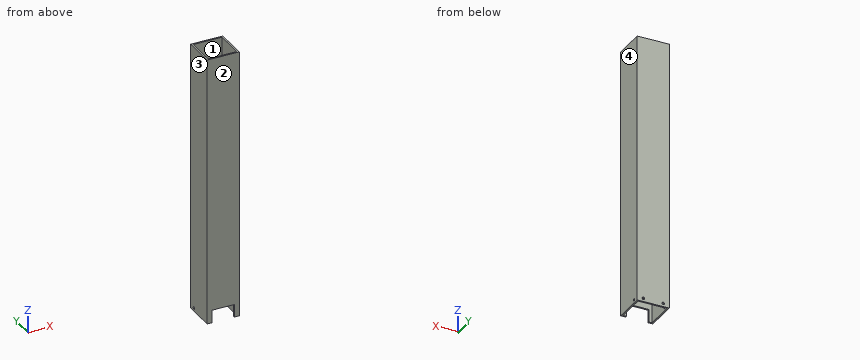
Autodesk Inventor part; units mm, degrees
ref_plane "YZ Plane" through (0, 0, 0) normal (1, 0, 0) x (0, 1, 0)
ref_plane "XZ Plane" through (0, 0, 0) normal (0, 1, 0) x (-1, 0, 0)
ref_plane "XY Plane" through (0, 0, 0) normal (0, 0, 1) x (1, 0, 0)
sketch "Sketch1" plane through (0, 0, 0) normal (0, 0, 1) x (1, 0, 0)
  line L0 (0, 0) -> (63.5, 0)
  line L1 (63.5, 0) -> (63.5, 63.5)
  line L2 (63.5, 63.5) -> (0, 63.5)
  line L3 (0, 63.5) -> (0, 0)
  line L4 (3.175, 60.325) -> (60.325, 60.325)
  line L5 (60.325, 60.325) -> (60.325, 3.175)
  line L6 (60.325, 3.175) -> (3.175, 3.175)
  line L7 (3.175, 3.175) -> (3.175, 60.325)
  dimension "d0" = 63.5
  dimension "d1" = 63.5
  dimension "d2" = 3.175
extrude "Extrusion1" add sketch "Sketch1" along normal blind 533.4
sketch "Sketch3" plane through (0, 63.5, 0) normal (0, 1, 0) x (1, 0, 0)
  line L0 (9.525, 0) -> (9.525, -25.4)
  line L1 (9.525, -25.4) -> (53.975, -25.4)
  line L2 (53.975, -25.4) -> (53.975, 0)
  line L3 (63.5, 0) -> (63.5, -533.4)
  line L4 (63.5, 0) -> (0, 0)
  line L5 (9.525, 0) -> (53.975, 0)
  line L6 (0, 0) -> (63.5, 0)
  line L7 (63.5, 0) -> (0, 0)
  line L8 (0, 0) -> (0, -533.4)
  line L9 (63.5, -533.4) -> (0, -533.4)
  line L10 (63.5, 0) -> (63.5, -533.4)
  dimension "d14" = 44.45
  dimension "d16" = 25.4
  dimension "d19" = 9.525
  dimension "d20" = 9.525
extrude "Extrusion2" cut sketch "Sketch3" against normal blind 63.5 contours L4 L2 L1 L0
sketch "Sketch5" plane through (0, 63.5, 533.4) normal (0, 1, 0) x (1, 0, 0)
  line L0 (53.975, 508) -> (9.525, 508)
  line L1 (53.975, 533.4) -> (53.975, 508)
  line L2 (9.525, 508) -> (9.525, 533.4)
  line L3 (53.975, 533.4) -> (9.525, 533.4)
  point P0 (0, 533.4)
extrude "Extrusion3" add sketch "Sketch5" against normal blind 3.175
sketch "Sketch6" plane through (0, 63.5, 0) normal (0, 1, 0) x (1, 0, 0)
  line L0 (0, 0) -> (0, -533.4)
  line L1 (63.5, 0) -> (63.5, -533.4)
  line L2 (63.5, 0) -> (0, 0)
  point P0 (12.192, -6.35)
  point P1 (51.308, -6.35)
  dimension "d23" = 12.192
  dimension "d24" = 12.192
  dimension "d25" = 6.35
hole "Hole2" at (12.192, 63.5, 6.35) at (51.308, 63.5, 6.35) direction (0, -1, 0) diameter 5.1562 depth 25.4 tip angle 118
sketch "Sketch7" plane through (63.5, 0, 0) normal (1, 0, 0) x (0, 0, -1)
  line L0 (0, 63.5) -> (-533.4, 63.5)
  line L1 (0, 0) -> (0, 63.5)
  point P0 (-6.35, 51.308)
  dimension "d33" = 12.192
  dimension "d34" = 6.35
hole "Hole3" at (63.5, 51.308, 6.35) direction (-1, 0, 0) diameter 5.1562 depth 76.2 tip angle 118
equation "\"d19\" = d20"
properties part number "TelescopeNewOuter" material "Aluminum 6061"
The listing builds one solid part. Answer for the finished solid, in the listing's coordinates (mm). Face numbers are marked on the shaded views. Round coordinates to 2 decimals unless told otherwise and drop trailing zeros. Write each loop counter-clockwise with the first axis right and the second up, starting at its lowest first coordinate (ties: lowest second). Pieces come first, ordered by that corner, then holes. Notation, with made-up numbers: (60.5, 15.5) -> (87.5, 15.5) arc R27 cw to (87.5, 43.5) -> close; hole circle Ø8 at (-11.75, 38.25). An arc over 180 degrees is marked (long way). Use CSV: the item, a comma, the result in double quotes. Start each with the question number.
(1) The mould has two halves that part along X. Classify the marked faces 1, 2, 3 and 4: released by +X, released by -X, zero draft, split by the parting line, or undercut.
(2) Consider L1, parallel to X at y = 61.65, z = 6.35; L2, parallel to Y at x = 60, z = 314 (3 decimals). Determine where each line is inside the solid, lowest interval first. Write a range as from..to.
(3) This flat-tipped pin is pushed along its axis until it touches: pin 1 (2.5 mm diameter, centred on x = 28.5, y = 1, fed in from -Z). Where does it stop, or does it pass through?
(4) Section B-B on z = 465 is taken. Give the vertices of the cut face in (x, y) (3 decimals), then the cut area to 3 significant figures.
(5) Section A-A on y = 31 is taken. Give the vertices of the cut face in (x, z) (3 decimals), then the cut area to 3 significant figures.
(6) Section C-C on x = 30 is taken. Give the vertices of the cut face in (y, z) (3 decimals), then the cut area to 3 significant figures.
A:
1,face 1,"undercut"
1,face 2,"zero draft"
1,face 3,"released by -X"
1,face 4,"released by +X"
2,L1,"x = 0..9.61, 14.77..48.73, 53.89..63.5"
2,L2,"y = 0..3.175, 60.325..63.5"
3,pin 1,"stops at z = 25.4"
4,outline,"(0, 0) -> (63.5, 0) -> (63.5, 63.5) -> (0, 63.5) -> close; hole (3.175, 3.175) -> (60.325, 3.175) -> (60.325, 60.325) -> (3.175, 60.325) -> close"
4,area,"766 mm²"
5,outline,"(0, 0) -> (3.175, 0) -> (3.175, 533.4) -> (0, 533.4) -> close; (60.325, 0) -> (63.5, 0) -> (63.5, 533.4) -> (60.325, 533.4) -> close"
5,area,"3,390 mm²"
6,outline,"(0, 25.4) -> (3.175, 25.4) -> (3.175, 533.4) -> (0, 533.4) -> close; (60.325, 0) -> (63.5, 0) -> (63.5, 533.4) -> (60.325, 533.4) -> close"
6,area,"3,310 mm²"
